```python
from build123d import *

# Parameters (mm, degrees)
SKETCH1_R           = 76.2
SKETCH1_R_2         = 15.875
BOSS_EXTRUDE1_DEPTH = 25.4
SKETCH2_R           = 31.75
BOSS_EXTRUDE2_DEPTH = 22.225


with BuildPart() as part:
    # Sketch1 → Boss-Extrude1 (new body)
    with BuildSketch(Plane.XY):
        Circle(SKETCH1_R)
        Circle(SKETCH1_R_2, mode=Mode.SUBTRACT)
    extrude(amount=BOSS_EXTRUDE1_DEPTH)

    # Sketch2 → Boss-Extrude2 (add)
    with BuildSketch(Plane.XY.offset(25.4)):
        Circle(SKETCH2_R)
    extrude(amount=BOSS_EXTRUDE2_DEPTH)


solid = part.part
```
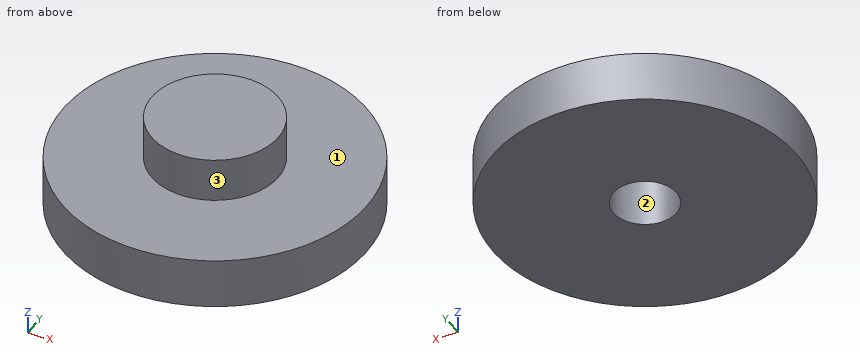
CAD build for the part. Positions are in the model's coordinates, mm. Face numbers are marked on the shaded views. Round coordinates to 2 decimals unless told otherwise and drop trailing zeros. Write each loop counter-clockwise with the first axis right and the second up, starting at its lowest first coordinate (ties: lowest second). Pieces come first, ordered by that corner, then holes. Notation, with made-up numbers: M 52,71 L 109,71 A24 ccw 109,105 Z; hole C 82.5,-24 d10. An arc over 180 degrees is marked long. One line per question, with ' | ' between items.
1. Pin check, flat tips, straight feed: pin 1 Ø12 at (x, z) = (27, 17.5) entering from +Y; pin 2 Ø16 at (x, y) = (-6.5, 6) entering from -Z; pin 3 Ø6 at (x, z) = (22.5, 27) entering from -Y; pin 4 Ø8 at (x, z) = (52, 15.5) entering from -Y. Stop position of each tip, or through.
Working result:
pin 1: y = 73.25 | pin 2: z = 0 | pin 3: y = -73.54 | pin 4: y = -59.18
2. Cut at D-D on z = 41. Write the cut outline in (x, y).
Working result:
outline: C 0,0 d63.5
3. Mould opens along Y. For the marked faces 1, 2 and 3 say: pulls with the +Y half, pulls with the -Y half, needs draft (parallel to the pull), parting line crosses it, or undercut.
Working result:
face 1: needs draft | face 2: undercut | face 3: parting line crosses it
4. Probe L1, parallel to Y at x = 0, z = 18.5 (3 decimals); L2, parallel to Z at x = -60.5, y = 19; L3, parallel to X at y = -13.5, z = 15. List the from-to ranges inside material, lowest first. Write a range as from..to.
Working result:
L1: -76.2..-15.875, 15.875..76.2 | L2: 0..25.4 | L3: -74.99..-8.35, 8.35..74.99
5. Cut at B-B on z = 23. Write the cut outline in (x, y) (3 decimals).
Working result:
outline: C 0,0 d152.4; hole C 0,0 d31.75
6. Cut at A-A on y = 0. Write the cut outline in (x, z) (3 decimals).
Working result:
outline: M -76.2,0 L -15.875,0 L -15.875,25.4 L 15.875,25.4 L 15.875,0 L 76.2,0 L 76.2,25.4 L 31.75,25.4 L 31.75,47.625 L -31.75,47.625 L -31.75,25.4 L -76.2,25.4 Z
